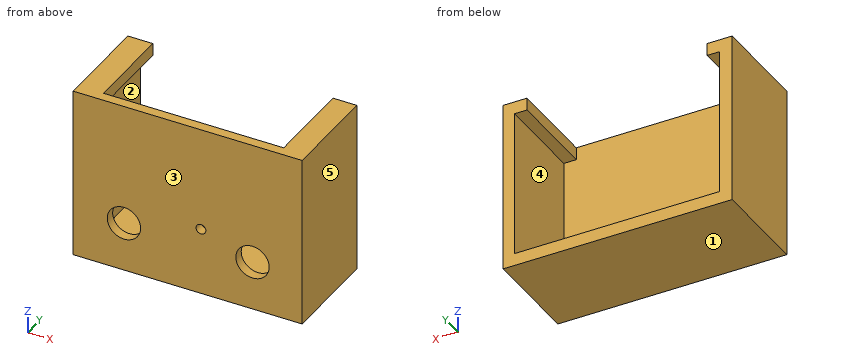
```python
from build123d import *

# Parameters (mm, degrees)
SKETCH1_W           = 23.33
SKETCH1_H           = 17.54
BOSS_EXTRUDE1_DEPTH = 10.16
SKETCH2_W           = 20.9
SKETCH2_H           = 15
CUT_EXTRUDE1_DEPTH  = 9.16
SKETCH3_R           = 1.7
SKETCH3_R_2         = 0.5
CUT_EXTRUDE2_DEPTH  = 31.591601789
SKETCH4_W           = 18.36
SKETCH4_H           = 12.01194936
CUT_EXTRUDE3_DEPTH  = 31.20310249


with BuildPart() as part:
    # Sketch1 → Boss-Extrude1 (new body)
    with BuildSketch(Plane(origin=(0, 0, 0), x_dir=(1, 0, 0), z_dir=(0, 1, 0))):
        with Locations((11.665, 8.77)):
            Rectangle(SKETCH1_W, SKETCH1_H)
    extrude(amount=BOSS_EXTRUDE1_DEPTH)

    # Sketch2 → Cut-Extrude1 (cut)
    with BuildSketch(Plane(origin=(0, 10.16, 0), x_dir=(1, 0, 0), z_dir=(0, 1, 0))):
        with Locations((11.72, 8.77)):
            Rectangle(SKETCH2_W, SKETCH2_H)
    extrude(amount=-CUT_EXTRUDE1_DEPTH, mode=Mode.SUBTRACT)

    # Sketch3 → Cut-Extrude2 (cut, through all)
    with BuildSketch(Plane(origin=(0, 1, 0), x_dir=(1, 0, 0), z_dir=(0, 1, 0))):
        with Locations(Location((5.17, 12.52, 0), (0, 0, 270))):
            Circle(SKETCH3_R)
        with Locations(Location((18.27, 12.52, 0), (0, 0, 270))):
            Circle(SKETCH3_R)
        with Locations(Location((13.015, 10.66, 0), (0, 0, 270))):
            Circle(SKETCH3_R_2)
    extrude(amount=-CUT_EXTRUDE2_DEPTH, mode=Mode.SUBTRACT)

    # Sketch4 → Cut-Extrude3 (cut, through all)
    with BuildSketch(Plane(origin=(0, 0, -1.27), x_dir=(-1, 0, 0), z_dir=(0, 0, -1))):
        with Locations((-11.72, 7.00597468)):
            Rectangle(SKETCH4_W, SKETCH4_H)
    extrude(amount=-CUT_EXTRUDE3_DEPTH, mode=Mode.SUBTRACT)


solid = part.part
```
The listing builds one solid part. Answer for the finished solid, in the listing's coordinates (mm). Face numbers are marked on the shaded views. A direction names the side the tool comes from. Give positions to 0.01 mm unless a question says otherwise; leave off trailing zeros. Order: outer loops, then holes, each group sorted by start corner. A loop starts at its lowest first (then second) coordinate and runs counter-clockwise, first axis right, second up.
Item 1: The part is cut by section D-D, the plane y = 5.25. Give the vertices of the cut face in (x, z).
From the geometry:
outline: (0, -17.54) - (23.33, -17.54) - (23.33, 0) - (20.9, 0) - (20.9, -1.27) - (22.17, -1.27) - (22.17, -16.27) - (1.27, -16.27) - (1.27, -1.27) - (2.54, -1.27) - (2.54, 0) - (0, 0) - close
Item 2: The part is cut by section B-B, the plane x = 18.27. Give the vertices of the cut face in (y, z), and give its area (3 significant figures).
From the geometry:
outline: (0, -17.54) - (10.16, -17.54) - (10.16, -16.27) - (1, -16.27) - (1, -14.22) - (0, -14.22) - close; (0, -10.82) - (1, -10.82) - (1, 0) - (0, 0) - close
area: 25.8 mm2
Item 3: Find the intervals of material crossed by probe 1 along X at (y, z) = (0.4, -12.52); probe 2 along X at (y, z) = (0.85, -10.66) (3 decimals); probe 3 along X at (y, z) = (3.75, -10.75), in increasing order.
From the geometry:
probe 1: x = 0 to 3.47, 6.87 to 16.57, 19.97 to 23.33
probe 2: x = 0 to 12.515, 13.515 to 23.33
probe 3: x = 0 to 1.27, 22.17 to 23.33
Item 4: The part is cut by section A-A, the plane z = -12.52. Give the vertices of the cut face in (x, y), and give its area (3 significant figures).
From the geometry:
outline: (0, 0) - (3.47, 0) - (3.47, 1) - (1.27, 1) - (1.27, 10.16) - (0, 10.16) - close; (6.87, 0) - (16.57, 0) - (16.57, 1) - (6.87, 1) - close; (19.97, 0) - (23.33, 0) - (23.33, 10.16) - (22.17, 10.16) - (22.17, 1) - (19.97, 1) - close
area: 38.8 mm2
Item 5: Given pin 1 Ø0.6 at (y, z) = (6, -0.5) entering from -X; pin 2 Ø5 at (x, z) = (15, -3) entering from +Y; pin 3 Ø4.5 at (x, y) = (11, 7.5) entering from +Z, each flat-ended and moving along its own axis, determine where each tip first touches the part or whether it passes through.
From the geometry:
pin 1: stops at x = 0
pin 2: stops at y = 1
pin 3: stops at z = -16.27
Item 6: For a pull along X with two mould halves and no side action, classify the marked faces 3, 4 and 5 as pulls with the +X half, pulls with the -X half, needs draft (parallel to the pull), parting line crosses it, or undercut.
From the geometry:
face 3: needs draft
face 4: undercut
face 5: pulls with the +X half
Item 7: Which of the six approach directions +Z, -Z, +X, -X, +Y, -Y give full straight-line access (tool end or side, diameter ignored) to the marked faces 1 and 2?
From the geometry:
face 1: -Z, +X, -X, +Y, -Y
face 2: +Y
Item 8: The part is cut by section C-C, the plane z = -1.75. Give the vertices of the cut face in (x, y).
From the geometry:
outline: (0, 0) - (23.33, 0) - (23.33, 10.16) - (22.17, 10.16) - (22.17, 1) - (1.27, 1) - (1.27, 10.16) - (0, 10.16) - close
